Could you check a few things on this model? Use its own coordinates, in mm. Coordinates: 2 decimals unless noted, no trailing zeros. Order: outer loops, then holes, each group sorted by start corner. A loop starts at its lowest first (then second) coordinate and runs counter-clockwise, first axis right, second up. Notation, with made-up numbers: M 54,-14.5 L 96,-14.5 A23 ccw 96,8.5 Z; hole C 41.5,-23.5 d5. An arc over 180 degrees is marked long. Write item = value, one per line. Start each with the question number.
from build123d import *

# Parameters (mm, degrees)
F0_W        = 8.89
F0_H        = 15.24
F1_DEPTH    = 10.16
F3_DEPTH    = 15.24
F4_T1_DEPTH = 36.2882991577
F5_T1_DEPTH = 36.5015311919
F6_T1_DEPTH = 33.8737387742


# Not quite as in the source:
# - a fillet or chamfer that OpenCascade refuses, or shapes differently, is made with other operations: its cross-section is extruded or revolved along the edge and cut away or added


with BuildPart() as f1:
    # F0 (on Top) → F1 (new body)
    with BuildSketch(Plane.XY):
        with Locations((-39.3944829702, 14.0595820769)):
            Rectangle(F0_W, F0_H)
    extrude(amount=F1_DEPTH)

    # F2 (on face) → F3 (join)
    with BuildSketch(Plane.XZ.offset(-6.4395820769)):
        Polygon((-43.8394829702, 10.16), (-34.9494829702, 10.16), (-39.3944829702, 16.349214409), align=None)
    extrude(amount=-F3_DEPTH)

    # F4: chamfer of 5.08 on 4 edges, made by hand

    # F4_s2 → F4_t1 (cut)
    with BuildSketch(Plane.XY.offset(-13.0641495789)):
        Polygon((-34.9494829702, 11.5195820769), (-40.0294829702, 6.4395820769), (-34.9494829702, 6.4395820769), align=None)
        Polygon((-43.8394829702, 11.5195820769), (-38.7594829702, 6.4395820769), (-43.8394829702, 6.4395820769), align=None)
        Polygon((-40.0294829702, 21.6795820769), (-34.9494829702, 16.5995820769), (-34.9494829702, 21.6795820769), align=None)
        Polygon((-38.7594829702, 21.6795820769), (-43.8394829702, 16.5995820769), (-43.8394829702, 21.6795820769), align=None)
    extrude(amount=F4_T1_DEPTH, mode=Mode.SUBTRACT)

    # F5: chamfer of 5.08 on 4 edges, made by hand

    # F5_s2 → F5_t1 (cut)
    with BuildSketch(Plane.XY.offset(-13.170765596)):
        Polygon((-34.9494829702, 11.5195820769), (-38.5415854186, 20.1916845253), (-34.9494829702, 16.5995820769), align=None)
        Polygon((-34.9494829702, 16.5995820769), (-38.5415854186, 7.9274796285), (-34.9494829702, 11.5195820769), align=None)
        Polygon((-40.2473805218, 7.9274796285), (-43.8394829702, 16.5995820769), (-43.8394829702, 11.5195820769), align=None)
        Polygon((-43.8394829702, 11.5195820769), (-40.2473805218, 20.1916845253), (-43.8394829702, 16.5995820769), align=None)
    extrude(amount=F5_T1_DEPTH, mode=Mode.SUBTRACT)

    # F6: chamfer of 5.08 on 1 edges, made by hand

    # F6_s2 → F6_t1 (cut)
    with BuildSketch(Plane(origin=(-11.3557841109, 27.415288012, -15.8117846218), x_dir=(0.9238795325, 0.3826834324, 0), z_dir=(0.3377298738, -0.8153520418, 0.4702548035))):
        Polygon((-34.1500159871, 18.9876434675), (-30.7922479627, 27.8797024774), (-34.1500159871, 24.0676434675), align=None)
    extrude(amount=F6_T1_DEPTH, mode=Mode.SUBTRACT)


solid = f1.part
(1) Will these pins go through, and if not, where does the flat tip stop? P1, Ø1.5, axis at y = 10.5, z = 6.5, coming from the +X side; P2, Ø6, axis at y = 19.5, z = 10.5, coming from the +X side.
(2) Please list where these lines run through material, in increasing order: probe 1 along Y at (x, z) = (-37, 11.5); probe 2 along Y at (x, z) = (-39, 9); probe 3 along X at (y, z) = (8.25, 13.75). Write a range as from..to.
(3) Imagine slicing it at C-C on x = -40. List the corners of the cut face in (y, z) for me.
(4) Imagine slicing it at A-A on z = 2.5. List the corners of the cut face in (x, y) for me.
(5) Imagine slicing it at B-B on y = 20. List the corners of the cut face in (x, z) for me, plus the area to 3 significant figures.
(6) Imagine slicing it at D-D on z = 9.75. List the corners of the cut face in (x, y) for me, plus the area to 3 significant figures.
Response:
q1.P1 = -37.17
q1.P2 = -37.01
q2.probe_1 = 11.65..16.47
q2.probe_2 = 7.47..20.65
q2.probe_3 = -38.86..-38.41
q3.outline = M 7.68,0 L 20.44,0 L 20.44,15.51 L 16.1,15.51 L 7.68,9.98 Z
q4.outline = M -42.79,14.06 L -40.25,7.93 L -39.39,7.07 L -38.54,7.93 L -36,14.06 L -38.54,20.19 L -39.39,21.04 L -40.25,20.19 Z
q5.outline = M -40.33,0 L -38.46,0 L -38.46,15.05 L -39.39,16.35 L -40.33,15.05 Z
q5.area = 29.3 mm2
q6.outline = M -41.94,16.11 L -40.1,7.78 L -39.39,7.07 L -38.54,7.93 L -36,14.06 L -38.54,20.19 L -39.39,21.04 L -40.25,20.19 Z
q6.area = 47.8 mm2
